from build123d import *

# Parameters (mm, degrees)
F1_DEPTH      = 30
F1_DEPTH_BACK = 30
F2_R          = 6
F3_DEPTH      = 10.001
F4_R          = 3
F5_W          = 8
F5_H          = 30
F6_DEPTH      = 100
F7_R          = 2


with BuildPart() as f1:
    # F0 (on Top) → F1 (new body, two sides)
    with BuildSketch(Plane.XY) as f1_sk:
        Polygon((-60, 10), (-60, 0), (60, 0), (60, 10), (28, 10), (28, 44), (23, 44), (23, 10), (-23, 10), (-23, 44), (-28, 44), (-28, 10), align=None)
    extrude(amount=F1_DEPTH)
    extrude(f1_sk.sketch, amount=-F1_DEPTH_BACK)

    # F2 (on face) → F3 (cut, through all)
    with BuildSketch(Plane(origin=(0, 10, 0), x_dir=(-1, 0, 0), z_dir=(0, 1, 0))):
        with Locations((44, 0)):
            Circle(F2_R)
        with Locations((-44, 0)):
            Circle(F2_R)
    extrude(amount=-F3_DEPTH, mode=Mode.SUBTRACT)

    # F4
    f4_edges = [f1.edges().sort_by_distance(p)[0] for p in [
        (28, 10, 0),
        (23, 10, 0),
        (-28, 10, 0),
        (-23, 10, 0),
    ]]
    fillet(f4_edges, radius=F4_R)

    # F5 (on face) → F6 (cut)
    with BuildSketch(Plane.YZ.offset(28)):
        with BuildLine():
            ThreePointArc((24, -15), (39, 0), (24, 15))
            Line((24, 15), (24, -15))
        make_face()
        with Locations((20, 0)):
            Rectangle(F5_W, F5_H)
    extrude(amount=-F6_DEPTH, mode=Mode.SUBTRACT)

    # F7
    f7_edges = [f1.edges().sort_by_distance(p)[0] for p in [
        (25.5, 16, -15),
        (-25.5, 16, -15),
        (25.5, 16, 15),
        (-25.5, 16, 15),
    ]]
    fillet(f7_edges, radius=F7_R)


solid = f1.part
Here's how the part is built. I have some questions about the finished solid (model axes, mm). A direction names the side the tool comes from. Coordinates: 2 decimals unless noted, no trailing zeros. Order: outer loops, then holes, each group sorted by start corner. A loop starts at its lowest first (then second) coordinate and runs counter-clockwise, first axis right, second up. Notation, with made-up numbers: M -33.5,39.5 L 20.5,39.5 A14 ccw 20.5,47.5 Z; hole C 65.25,29.25 d2. An arc over 180 degrees is marked long. Answer as CSV lines item,"result".
Item 1: If I drill on line 1 (X direction, y = 17.5, z = 23.5); line 2 (Z direction, x = 44, y = 6.25); line 3 (Y direction, x = -44.5, z = -21.5), over which ranges is the centre line in solid material (lowest first)?
Results found:
line 1,"-28 to -23, 23 to 28"
line 2,"-30 to -6, 6 to 30"
line 3,"0 to 10"
Item 2: Imagine slicing it at B-B on y = 11.5. Write out the boundary of the cut face in (x, z), plus the area to 3 significant figures.
Results found:
outline,"M -28.4,-30 L -22.6,-30 L -22.6,30 L -28.4,30 Z; M 22.6,-30 L 28.4,-30 L 28.4,30 L 22.6,30 Z"
area,"696 mm2"
Item 3: Imagine slicing it at C-C on z = 0. Give the number of separate pieces and of enclosed holes in the cut face, plus the area to 3 significant figures.
Results found:
separate pieces,"5"
enclosed holes,"0"
area,"1,080 mm2"
Item 4: We'd pull the mould along Z, two halves only. Please class faces 1 (the face through (-23, 39, 7)), 2 (the face through (-25, 21, 15)): +Z half, -Z half, draft (parallel to the pull), parting line (faces both ways), or undercut.
Results found:
face 1,"draft"
face 2,"undercut"
Item 5: On a 3-axis mill with a long thin cutter (end or side, diameter ignored), from which of +Z, -Z, +X, -X, +Y, -Y can I reach the whole of each face in a straight line? I mean faces 3 (the face through (0, 10, 0)), 4 (the face through (-25, 21, -15)), 5 (the face through (28, 39, 7)). Say none if no direction works.
Results found:
face 3,"+Z, -Z, +Y"
face 4,"+X, -X"
face 5,"+Z, -Z, +X, +Y"
Item 6: For pin 1 (14.5 mm diameter, centred on x = -39.5, z = 5, fed in from +Y); pin 2 (12 mm diameter, centred on y = 17.5, z = 16, fed in from +X); pin 3 (2 mm diameter, centred on y = 21, z = -20.5, fed in from +X), each with a flat end and sliding along its axis, tell me the tip position at first contact or that it passes through.
Results found:
pin 1,"y = 10"
pin 2,"x = 28.4"
pin 3,"x = 28"
Item 7: Imagine slicing it at D-D on y = 28. Write out the boundary of the cut face in (x, z).
Results found:
outline,"M -28,-30 L -23,-30 L -23,-14.46 L -28,-14.46 Z; M -28,14.46 L -23,14.46 L -23,30 L -28,30 Z; M 23,-30 L 28,-30 L 28,-14.46 L 23,-14.46 Z; M 23,14.46 L 28,14.46 L 28,30 L 23,30 Z"
Item 8: Imagine slicing it at A-A on x = 44. Write out the boundary of the cut face in (y, z), plus the area to 3 significant figures.
Results found:
outline,"M 0,-30 L 10,-30 L 10,-6 L 0,-6 Z; M 0,6 L 10,6 L 10,30 L 0,30 Z"
area,"480 mm2"
